Source: three-view drawing plus pictorial views. Frame: mm from the lowest corner of the part. Round coordinates to 2 decimals unless told otherwise and drop trailing zeros. Order: outer loops, then holes, each group sorted by start corner. A loop starts at its lowest first (then second) coordinate and runs counter-clockwise, first axis right, second up. Notation, with made-up numbers: (28.5, 13.25) -> (62.5, 13.25) arc R34 cw to (62.5, 52.25) -> close; hole circle Ø2 at (23.5, 49). An arc over 180 degrees is marked (long way). Use a Markdown table: item, result.
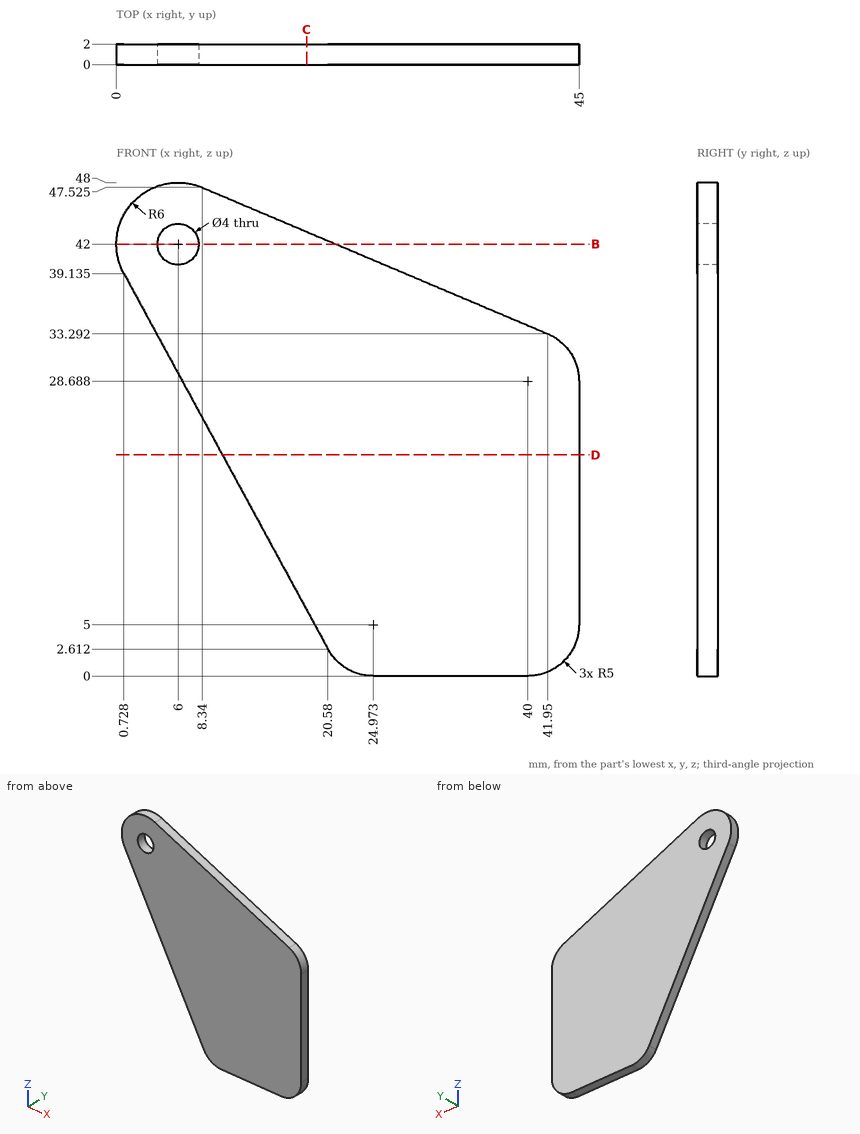
1) Cut plane D-D on z = 21.5. Return loops of the section in (x, y).
Results found:
| item | result |
|---|---|
| outline | (10.31, 0) -> (45, 0) -> (45, 2) -> (10.31, 2) -> close |
2) Cut plane C-C on x = 18.5. Return loops of the section in (y, z).
Results found:
| item | result |
|---|---|
| outline | (0, 6.44) -> (2, 6.44) -> (2, 43.22) -> (0, 43.22) -> close |
3) Cut plane B-B on z = 42. Return loops of the section in (x, y).
Results found:
| item | result |
|---|---|
| outline | (0, 0) -> (4, 0) -> (4, 2) -> (0, 2) -> close; (8, 0) -> (21.39, 0) -> (21.39, 2) -> (8, 2) -> close |
4) Line query: L1, parallel to Z at x = 7, y = 0.25 (1 decimal); L2, parallel to Z at x = 4.5, y = 0.8 (1 decimal); L3, parallel to X at y = 1.6, z = 28. Output: solid intervals per line, ascending. Write a range as [from, to].
Results found:
| item | result |
|---|---|
| L1 | z = [27.6, 40.3], [43.7, 47.9] |
| L2 | z = [32.2, 40.7], [43.3, 47.8] |
| L3 | x = [6.78, 45] |
